from build123d import *

# Parameters (mm, degrees)
BOSS_EXTRUDE1_DEPTH = 2.3
SKETCH5_W           = 65
SKETCH5_H           = 45
CUT_EXTRUDE1_DEPTH  = 3.3
FILLET1_R           = 2
SKETCH7_W           = 2.3
SKETCH7_H           = 10
SKETCH7_W_2         = 10
SKETCH7_H_2         = 2.3
CUT_EXTRUDE2_DEPTH  = 3.3
SKETCH8_R           = 1
CUT_EXTRUDE3_DEPTH  = 3.3
SKETCH10_R          = 1.15
CUT_EXTRUDE4_DEPTH  = 3.3
SKETCH11_W          = 8
SKETCH11_H          = 3
CUT_EXTRUDE5_DEPTH  = 10
SKETCH12_R          = 1
CUT_EXTRUDE6_DEPTH  = 10


with BuildPart() as part:
    # Sketch1 → Boss-Extrude1 (new body)
    with BuildSketch(Plane.XY):
        Polygon((0, 0), (100, 0), (100, -57), (77, -57), (77, -90), (23, -90), (23, -57), (0, -57), align=None)
    extrude(amount=BOSS_EXTRUDE1_DEPTH)

    # Sketch5 → Cut-Extrude1 (cut, through all)
    with BuildSketch(Plane.XY.offset(2.3)):
        with Locations((50, -29.5)):
            Rectangle(SKETCH5_W, SKETCH5_H)
    extrude(amount=-CUT_EXTRUDE1_DEPTH, mode=Mode.SUBTRACT)

    # Fillet1
    fillet1_edges = [part.edges().sort_by_distance(p)[0] for p in [
        (82.5, -7, 1.15),
        (82.5, -52, 1.15),
        (17.5, -52, 1.15),
        (17.5, -7, 1.15),
    ]]
    fillet(fillet1_edges, radius=FILLET1_R)

    # Sketch7 → Cut-Extrude2 (cut, through all)
    with BuildSketch(Plane.XY.offset(2.3)):
        with Locations((91, -15)):
            Rectangle(SKETCH7_W, SKETCH7_H)
        with Locations((91, -45)):
            Rectangle(SKETCH7_W, SKETCH7_H)
        with Locations((9, -15)):
            Rectangle(SKETCH7_W, SKETCH7_H)
        with Locations((9, -45)):
            Rectangle(SKETCH7_W, SKETCH7_H)
        with Locations((37.5, -86)):
            Rectangle(SKETCH7_W_2, SKETCH7_H_2)
        with Locations((62.5, -86)):
            Rectangle(SKETCH7_W_2, SKETCH7_H_2)
    extrude(amount=-CUT_EXTRUDE2_DEPTH, mode=Mode.SUBTRACT)

    # Sketch8 → Cut-Extrude3 (cut, through all)
    with BuildSketch(Plane.XY.offset(2.3)):
        with Locations((15.5, -3)):
            Circle(SKETCH8_R)
        with Locations((84.5, -3)):
            Circle(SKETCH8_R)
    extrude(amount=-CUT_EXTRUDE3_DEPTH, mode=Mode.SUBTRACT)

    # Sketch10 → Cut-Extrude4 (cut, through all)
    with BuildSketch(Plane.XY.offset(2.3)):
        with Locations((49.9996888, -71.875)):
            Circle(SKETCH10_R)
        with Locations((31.2496888, -61.7)):
            Circle(SKETCH10_R)
        with Locations((68.7496888, -61.7)):
            Circle(SKETCH10_R)
        with Locations((31.2496888, -82.05)):
            Circle(SKETCH10_R)
        with Locations((68.7496888, -82.05)):
            Circle(SKETCH10_R)
    extrude(amount=-CUT_EXTRUDE4_DEPTH, mode=Mode.SUBTRACT)

    # Sketch11 → Cut-Extrude5 (cut)
    with BuildSketch(Plane.XY.offset(2.3)):
        with Locations((4, -1.5)):
            Rectangle(SKETCH11_W, SKETCH11_H)
        with Locations((96, -1.5)):
            Rectangle(SKETCH11_W, SKETCH11_H)
    extrude(amount=-CUT_EXTRUDE5_DEPTH, mode=Mode.SUBTRACT)

    # Sketch12 → Cut-Extrude6 (cut)
    with BuildSketch(Plane.XY.offset(2.3)):
        with Locations((4, -11)):
            Circle(SKETCH12_R)
        with Locations((96, -11)):
            Circle(SKETCH12_R)
    extrude(amount=-CUT_EXTRUDE6_DEPTH, mode=Mode.SUBTRACT)


solid = part.part
The listing builds one solid part. Answer for the finished solid, in the listing's coordinates (mm). A direction names the side the tool comes from. Give positions to 0.01 mm unless a question says otherwise; leave off trailing zeros. Loops run counter-clockwise (first coordinate to the right, second up) from the corner with the lowest first, then second, coordinate; pieces in that order, holes last.
Item 1: A tool of negligible diameter and unlimited length cuts with its end or side. For faces 1 (the flat face through (96, -3, 1)), 2 (the flat face through (62, -84.85, 1)), 3 (the flat face through (23, -74, 1)), from which of +Z, -Z, +X, -X, +Y, -Y can it reach the whole face along a straight path? Write none if from no direction.
Derived:
face 1: +Z, -Z, +X, +Y
face 2: +Z, -Z
face 3: +Z, -Z, -X, -Y
Item 2: Find the intervals of material crossed by line 1 along Y through (x, z) = (9.5, 2); line 2 along X through (y, z) = (-24.5, 0.8); line 3 along Y through (x, z) = (44.5, 1.6), in increasing order.
Derived:
line 1: y = -57 to -50, -40 to -20, -10 to 0
line 2: x = 0 to 17.5, 82.5 to 100
line 3: y = -90 to -52, -7 to 0
Item 3: A cutting plane is placed at B-B (x = 26). Give the vertices of the cut face in (y, z).
Derived:
outline: (-90, 0) - (-52, 0) - (-52, 2.3) - (-90, 2.3) - close; (-7, 0) - (0, 0) - (0, 2.3) - (-7, 2.3) - close
Item 4: Determine the mould class of faces 4 (the flat face through (49, 0, 1)), 5 (the cylindrical face through (67.902, -60.923, 1.166)), 6 (the flat face through (100, -30, 1)) for opening direction X: +X half, -X half, draft (parallel to the pull), parting line (faces both ways), or undercut.
Derived:
face 4: draft
face 5: undercut
face 6: +X half
Item 5: A cutting plane is placed at D-D (z = 1.95). Give the number of separate pieces and of enclosed holes in the cut face, then the cut area to 3 significant figures.
Derived:
separate pieces: 1
enclosed holes: 16
area: 4,340 mm2
Item 6: A cutting plane is placed at A-A (y = -82.05). Give the vertices of the cut face in (x, z), then the cut area to 3 significant figures.
Derived:
outline: (23, 0) - (30.1, 0) - (30.1, 2.3) - (23, 2.3) - close; (32.4, 0) - (67.6, 0) - (67.6, 2.3) - (32.4, 2.3) - close; (69.9, 0) - (77, 0) - (77, 2.3) - (69.9, 2.3) - close
area: 114 mm2
Item 7: Each of these flat-tipped pins is pushed along its axis until it touches: pin 1 Ø0.7 at (x, z) = (5, 1.5) entering from +Y; pin 2 Ø0.7 at (y, z) = (-15.5, 1) entering from -X; pin 3 Ø1.2 at (y, z) = (-2, 1.5) entering from -X; pin 4 Ø1.2 at (x, z) = (13, 1.5) entering from -Y. Where does it stop, or does it pass through?
Derived:
pin 1: stops at y = -3
pin 2: stops at x = 0
pin 3: stops at x = 8
pin 4: stops at y = -57
Item 8: A cutting plane is placed at C-C (x = 87). Give the vertices of the cut face in (y, z), then the cut area to 3 significant figures.
Derived:
outline: (-57, 0) - (0, 0) - (0, 2.3) - (-57, 2.3) - close
area: 131 mm2
